Design review of the part shown in the three views and the two pictorial views. Dimensions are in mm from the part's minimum x, y and z. A direction names the side the tool comes from. Round coordinates to 2 decimals unless told otherwise and drop trailing zeros. Loops run counter-clockwise (first coordinate to the right, second up) from the corner with the lowest first, then second, coordinate; pieces in that order, holes last.
1) Take a section at D-D (z = 24). State the section outline as (x, y) points.
2) Mouldability with a two-part tool opening along Z and no side actions: class the marked faces 1, 2 and 3 as pulls with the +Z half, pulls with the -Z half, needs draft (parallel to the pull), parting line crosses it, or undercut.
3) Take a section at A-A (z = 32.75). State the section outline as (x, y) points, then the cut area to 3 significant figures.
4) Take a section at B-B (x = 32.75). State the section outline as (y, z) points, then the cut area to 3 significant figures.
5) Tool access review of the marked faces 4 and 5: name each direction out of +Z, -Z, +X, -X, +Y, -Y from which nothing blocks a thin tool from reaching the whole face with its end or side.
6) Take a section at C-C (y = 6.5). State the section outline as (x, z) points.
7) Wall thickness on L1, parallel to X at y = 1.75, z = 32.75; L2, parallel to Y at x = 57.5, z = 26.5; L3, parallel to Z at x = 15, y = 2.25: over which ranges is each line inside the solid? List them lowest first.
8) Insertion check: pin 1 (3 mm diameter, centred on x = 23, z = 22.5, fed in from -Y); pin 2 (1 mm diameter, centred on y = 8, z = 44, fed in from -X); pin 3 (1 mm diameter, centred on y = 4.5, z = 16.5, fed in from -X). Each pin has a flat end and moves straight along its axis. Give the tip position at first contact, or say it passes through.
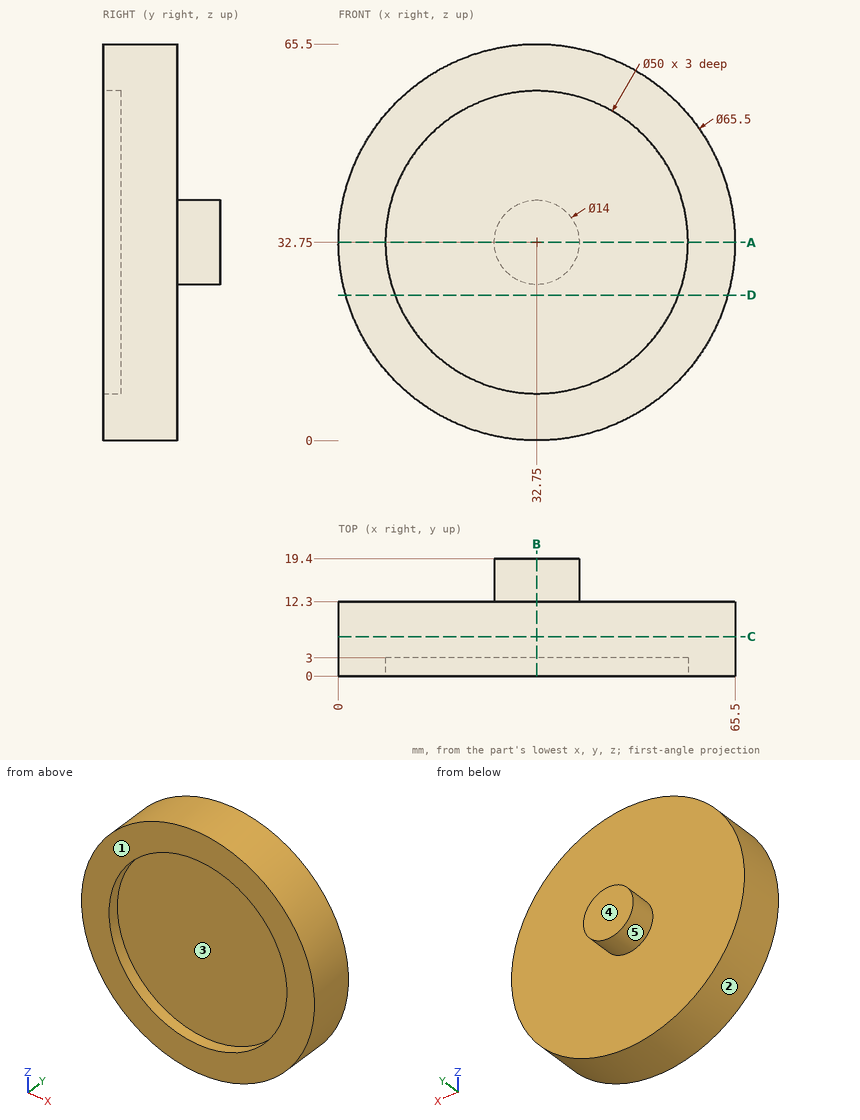
Response:
1. outline: (1.19, 0) - (9.33, 0) - (9.33, 3) - (56.17, 3) - (56.17, 0) - (64.31, 0) - (64.31, 12.3) - (1.19, 12.3) - close
2. face 1: needs draft
2. face 2: parting line crosses it
2. face 3: undercut
3. outline: (0, 0) - (7.75, 0) - (7.75, 3) - (57.75, 3) - (57.75, 0) - (65.5, 0) - (65.5, 12.3) - (39.75, 12.3) - (39.75, 19.4) - (25.75, 19.4) - (25.75, 12.3) - (0, 12.3) - close
3. area: 755 mm2
4. outline: (0, 0) - (12.3, 0) - (12.3, 25.75) - (19.4, 25.75) - (19.4, 39.75) - (12.3, 39.75) - (12.3, 65.5) - (0, 65.5) - (0, 57.75) - (3, 57.75) - (3, 7.75) - (0, 7.75) - close
4. area: 755 mm2
5. face 4: +Z, -Z, +X, -X, +Y
5. face 5: +Y
6. outline: circle Ø65.5 at (32.75, 32.75)
7. L1: x = 0 to 7.75, 57.75 to 65.5
7. L2: y = 0 to 12.3
7. L3: z = 5.23 to 15.14, 50.36 to 60.27
8. pin 1: stops at y = 3
8. pin 2: stops at x = 1.81
8. pin 3: stops at x = 4.04
